```python
from build123d import *

# Parameters (mm, degrees)
F0_W     = 58
F0_H     = 52
F0_W_2   = 30
F0_H_2   = 20
F1_DEPTH = 2
F2_D     = 3.3
F3_D     = 4.4


with BuildPart() as f1:
    # F0 (on Top) → F1 (new body)
    with BuildSketch(Plane.XY):
        Rectangle(F0_W, F0_H)
        with Locations((-2, 0)):
            Rectangle(F0_W_2, F0_H_2, mode=Mode.SUBTRACT)
    extrude(amount=F1_DEPTH)

    # F2 (through all)
    with Locations(Plane(origin=(0, 0, 0), x_dir=(1, 0, 0), z_dir=(0, 0, -1))):
        with Locations((-19.5, 15), (-25, 22.5), (-19.5, -15), (-25, -22.5), (15.5, 15), (15.5, -15), (25, -22.5), (25, 22.5)):
            Hole(F2_D / 2)

    # F3 (through all)
    with Locations(Plane(origin=(0, 0, 0), x_dir=(1, 0, 0), z_dir=(0, 0, -1))):
        with Locations((-24.5, 8), (-24.5, -8), (23.5, 8), (23.5, -8)):
            Hole(F3_D / 2)


solid = f1.part
```
Part model, mm, in its own coordinate system. A direction names the side the tool comes from. Round coordinates to 2 decimals unless told otherwise and drop trailing zeros. Write each loop counter-clockwise with the first axis right and the second up, starting at its lowest first coordinate (ties: lowest second). Pieces come first, ordered by that corner, then holes. Notation, with made-up numbers: (84.5, 82.25) -> (142.5, 82.25) arc R22 ccw to (142.5, 120.25) -> close; hole circle Ø10 at (19.25, 73.5). An arc over 180 degrees is marked (long way). Return JSON: item names as keys, results as strings. Group by question number.
Q1. Saw through at C-C on y = 8. Write the cut outline in (x, z).
Q2. Pin check, flat tip, straight feed: pin 1 (8 mm diameter, centred on x = 21, y = -9.5, fed in from -Z). Stop position of the tip, or through.
Q3. Saw through at D-D on z = 0.35. State how many separate pieces and enclosed holes the cut face has, plus the area to 3 significant figures.
Q4. Probe L1, parallel to X at y = -22.5, z = 0.85; L2, parallel to X at y = 2, z = 0.65; L3, parallel to Y at x = -14.5, z = 1.3. List the from-to ranges inside material, lowest first. Write a range as [from, to].
Q5. Which spindle directions (+Z, -Z, +X, -X, +Y, -Y) get a long thin tool onto all of the face, cutting with end or side? Do faces 1 (the flat face through (0, 12, 2)), 2 (the flat face through (-2, -10, 1)). Say none if no direction does.
Q6. Saw through at A-A on y = -15. Write the cut outline in (x, z), plus the area to 3 significant figures.
Q7. Saw through at B-B on x = -19.5. Write the cut outline in (y, z).
Q8. Mould opens along X. For faces 3 (the cylindrical face through (26.216, -23.615, 1.014)), 4 (the flat face through (-29, 0, 1)), 5 (the flat face through (0, 12, 0)) say: pulls with the +X half, pulls with the -X half, needs draft (parallel to the pull), parting line crosses it, or undercut.
Answer:
{
 "1": {"outline": "(-29, 0) -> (-26.7, 0) -> (-26.7, 2) -> (-29, 2) -> close; (-22.3, 0) -> (-17, 0) -> (-17, 2) -> (-22.3, 2) -> close; (13, 0) -> (21.3, 0) -> (21.3, 2) -> (13, 2) -> close; (25.7, 0) -> (29, 0) -> (29, 2) -> (25.7, 2) -> close"},
 "2": {"pin 1": "z = 0"},
 "3": {"separate pieces": "1", "enclosed holes": "13", "area": "2,290 mm2"},
 "4": {"L1": "[-29, -26.65], [-23.35, 23.35], [26.65, 29]", "L2": "[-29, -17], [13, 29]", "L3": "[-26, -10], [10, 26]"},
 "5": {"face 1": "+Z, +X, -X, +Y, -Y", "face 2": "+Z, -Z"},
 "6": {"outline": "(-29, 0) -> (-21.15, 0) -> (-21.15, 2) -> (-29, 2) -> close; (-17.85, 0) -> (13.85, 0) -> (13.85, 2) -> (-17.85, 2) -> close; (17.15, 0) -> (29, 0) -> (29, 2) -> (17.15, 2) -> close", "area": "103 mm2"},
 "7": {"outline": "(-26, 0) -> (-16.65, 0) -> (-16.65, 2) -> (-26, 2) -> close; (-13.35, 0) -> (13.35, 0) -> (13.35, 2) -> (-13.35, 2) -> close; (16.65, 0) -> (26, 0) -> (26, 2) -> (16.65, 2) -> close"},
 "8": {"face 3": "undercut", "face 4": "pulls with the -X half", "face 5": "needs draft"}
}
